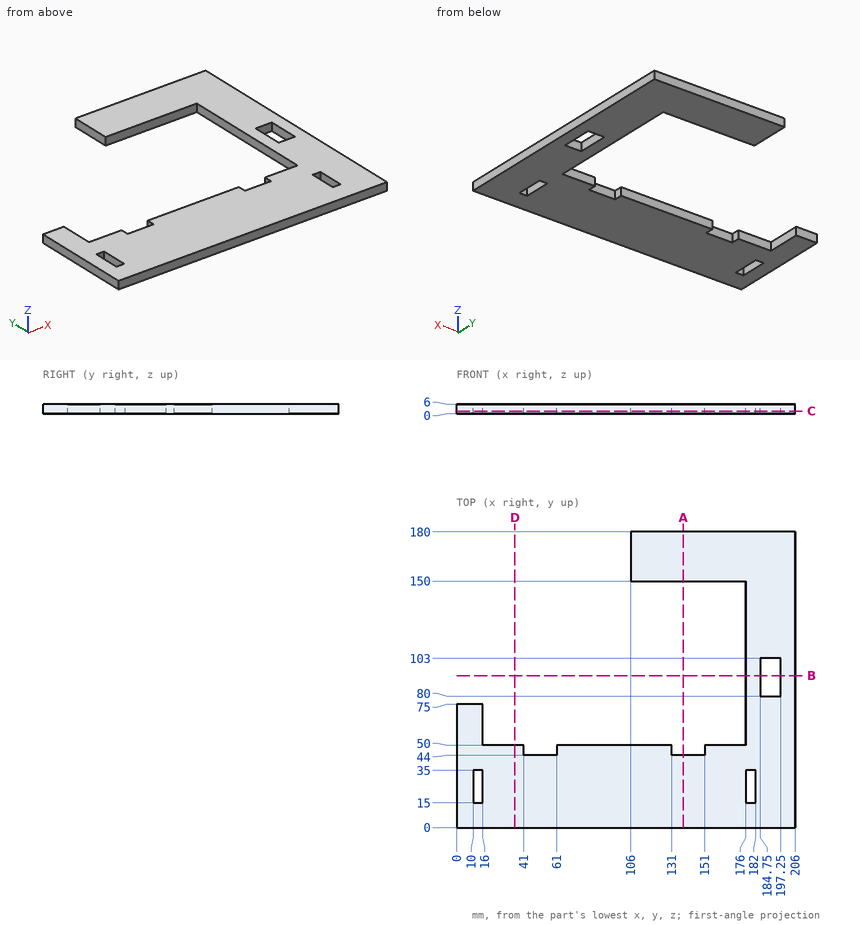
Design review of the part shown in the three views and the two pictorial views. Dimensions are in mm from the part's minimum x, y and z. Give positions to 0.01 mm unless a question says otherwise; leave off trailing zeros. Loops run counter-clockwise (first coordinate to the right, second up) from the corner with the lowest first, then second, coordinate; pieces in that order, holes last. Notation, with made-up numbers: (45, -23) -> (51, -23) arc R35 cw to (51, 15) -> close; hole circle Ø5 at (46, 13.25). An arc over 180 degrees is marked (long way). One line per item, written item: value.
Q1. We need section D-D on x = 35.5. Give the boundary of the cut face in (y, z), and give its area (3 significant figures).
Numbers:
outline: (0, 0) -> (50, 0) -> (50, 6) -> (0, 6) -> close
area: 300 mm^2
Q2. We need section B-B on y = 92.5. Give the boundary of the cut face in (x, z), and give its area (3 significant figures).
Numbers:
outline: (176, 0) -> (184.75, 0) -> (184.75, 6) -> (176, 6) -> close; (197.25, 0) -> (206, 0) -> (206, 6) -> (197.25, 6) -> close
area: 105 mm^2
Q3. For L1, parallel to X at y = 25.5, z = 5; L2, parallel to X at y = 46, z = 2.8; L3, parallel to Y at x = 128, z = 1.95, list the stretches that pass through material, from the lowest coordinate up.
Numbers:
L1: x = 0 to 10, 16 to 176, 182 to 206
L2: x = 0 to 41, 61 to 131, 151 to 206
L3: y = 0 to 50, 150 to 180
Q4. We need section C-C on z = 1.65. Give the number of separate pieces and of enclosed holes in the cut face, and give its area (3 significant figures).
Numbers:
separate pieces: 1
enclosed holes: 3
area: 15,900 mm^2
Q5. We need section A-A on x = 138. Give the boundary of the cut face in (y, z), and give its area (3 significant figures).
Numbers:
outline: (0, 0) -> (44, 0) -> (44, 6) -> (0, 6) -> close; (150, 0) -> (180, 0) -> (180, 6) -> (150, 6) -> close
area: 444 mm^2
Q6. For pin 1 Ø2 at (x, z) = (62.5, 0.5) entering from +Y, flat-tipped, find the tip position at first contact; note if it passes through.
Numbers:
pin 1: stops at y = 50
